Check sheet for the modelled part. Datum: model origin and axes. Units: mm. A direction names the side the tool comes from. Give positions to 0.01 mm unless a question says otherwise; leave off trailing zeros. Write each loop counter-clockwise with the first axis right and the second up, starting at its lowest first coordinate (ties: lowest second). Pieces come first, ordered by that corner, then holes. Notation, with made-up numbers: (30.5, 12) -> (41.5, 12) arc R24 ccw to (41.5, 22) -> close; hole circle Ø4 at (-13.75, 41.5). An arc over 180 degrees is marked (long way). Use a Markdown table: item, result. Add a question column.
1. Set-up check for faces 1 (the flat face through (5, 23, -37.008)), 2 (the flat face through (-1, -32.004, -31)): record each of +Z, -Z, +X, -X, +Y, -Y from which the full face is reachable in a straight line by a thin tool's end or side.
2. Scan lines: probe 1 along Y at (x, z) = (0, -49); probe 2 along X at (y, z) = (-7, -49.5); probe 3 along X at (y, z) = (0, -50). Record each from-to range of solid material in increasing order. Write a range as [from, to].
3. Cross-section at D-D (x = 31). Enter the section's corners in (y, z), then the cut area to 3 significant figures.
4. Cross-section at A-A (z = -51). Enter the section's corners in (x, y), then the cut area to 3 significant figures.
5. Cross-section at B-B (x = 0). Enter the section's corners in (y, z), then the cut area to 3 significant figures.
6. Release check for a two-part mould opening along X. For faces 3 (the flat face through (-43.002, -8, -38)), 4 (the flat face through (-1, -29, 0)), 5 (the cylindrical face through (-3.03, 23.07, -49.27)), 6 (the cylindrical face through (-33.39, -0.95, -40.33)) record: released by +X, released by -X, zero draft, split by the parting line, or undercut.
7. Cross-section at C-C (y = 0). Enter the section's corners in (x, z).
8. Gauge pin test, flat ends, axial feed: P1, Ø12, axis at x = -21.5, z = -25.5, coming from the +Y side; P2, Ø6, axis at x = 10.5, z = -24.5, coming from the +Y side; P3, Ø11, axis at x = 32.49, z = -47.02, coming from the -Y side. Record the tip position at first contact, or that the pin passes through.
from build123d import *

# Parameters (mm, degrees)
SKETCH1_W          = 86.0044
SKETCH1_H          = 62.992
SKETCH1_R          = 23.2665
EXTRUDE1_DEPTH     = 62.992
CUT_EXTRUDE1_DEPTH = 87.0044
SKETCH3_R          = 25.4
CUT_EXTRUDE2_DEPTH = 37.0078
FILLET1_R          = 1.524
HOLE1_D            = 13.4874
HOLE1_DEPTH        = 62.992


with BuildPart() as part:
    # Sketch1 → Extrude1 (new body)
    with BuildSketch(Plane.XY):
        with Locations((0, -0.508)):
            Rectangle(SKETCH1_W, SKETCH1_H)
        Circle(SKETCH1_R, mode=Mode.SUBTRACT)
    extrude(amount=-EXTRUDE1_DEPTH)

    # Sketch2 → Cut-Extrude1 (cut, through all)
    with BuildSketch(Plane(origin=(43.0022, 0, 0), x_dir=(0, 0, -1), z_dir=(1, 0, 0))):
        Polygon((0, 30.988), (37.592, 30.988), (0, -25.5016), align=None)
    extrude(amount=-CUT_EXTRUDE1_DEPTH, mode=Mode.SUBTRACT)

    # Sketch3 → Cut-Extrude2 (cut)
    with BuildSketch(Plane(origin=(0, 0, 0), x_dir=(-1, 0, 0), z_dir=(0, 0, -1))):
        with Locations(Location((0, 0, 0), (0, 0, 180))):  # turned: the seam where the file's is
            Circle(SKETCH3_R)
    extrude(amount=CUT_EXTRUDE2_DEPTH, mode=Mode.SUBTRACT)

    # Fillet1
    fillet1_edges = [part.edges().sort_by_distance(p)[0] for p in [
        (-25.4, 0, -37.0078),
    ]]
    fillet(fillet1_edges, radius=FILLET1_R)

    # Hole1
    with Locations(Plane(origin=(0, 30.988, 0), x_dir=(-1, 0, 0), z_dir=(0, 1, 0))):
        with Locations((32.512, -47.0154), (-32.4866, -47.0154)):
            Hole(HOLE1_D / 2, depth=HOLE1_DEPTH)

    # Sketch6 → Cut-Revolve1 (revolve, cut)
    with BuildSketch(Plane(origin=(0, 0, 0), x_dir=(-1, 0, 0), z_dir=(0, 1, 0)), mode=Mode.PRIVATE) as cut_revolve1_sk:
        Polygon((25.4, -34.671), (25.4, -35.433), (25.781, -35.052), align=None)
        Polygon((23.2665, -61.8745), (23.2665, -62.992), (24.384, -62.992), align=None)
    revolve(cut_revolve1_sk.sketch.rotate(Axis((0, 0, 17.508123997), (0, 0, -1)), 180), axis=Axis((0, 0, 17.508123997), (0, 0, -1)), mode=Mode.SUBTRACT)  # turned: the seam where the file's is


solid = part.part
Worked answers:
| question | item | result |
|---|---|---|
| 1 | face 1 | +Z |
| 1 | face 2 | +Z, -Z, +X, -X, -Y |
| 2 | probe 1 | y = [-32, -23.27], [23.27, 30.99] |
| 2 | probe 2 | x = [-43, -38.78], [-26.24, -22.19], [22.19, 26.22], [38.76, 43] |
| 2 | probe 3 | x = [-43, -38.56], [-26.46, -23.27], [23.27, 26.44], [38.53, 43] |
| 3 | outline | (-32, -62.99) -> (30.99, -62.99) -> (30.99, -53.59) -> (-32, -53.59) -> close; (-32, -40.44) -> (30.99, -40.44) -> (30.99, -37.59) -> (-25.5, 0) -> (-32, 0) -> close |
| 3 | area | 2,080 mm² |
| 4 | outline | (-43, -32) -> (-37.95, -32) -> (-37.95, 30.99) -> (-43, 30.99) -> close; (-27.07, -32) -> (27.05, -32) -> (27.05, 30.99) -> (-27.07, 30.99) -> close; (37.93, -32) -> (43, -32) -> (43, 30.99) -> (37.93, 30.99) -> close; hole circle Ø46.53 at (0, 0) |
| 4 | area | 2,350 mm² |
| 5 | outline | (-32, -62.99) -> (-24.38, -62.99) -> (-23.27, -61.87) -> (-23.27, -37.01) -> (-23.88, -37.01) arc R1.52 cw to (-25.4, -35.48) -> (-25.4, -35.43) -> (-25.78, -35.05) -> (-25.4, -34.67) -> (-25.4, -0.07) -> (-25.5, 0) -> (-32, 0) -> close; (23.27, -61.87) -> (24.38, -62.99) -> (30.99, -62.99) -> (30.99, -37.59) -> (25.4, -33.87) -> (25.4, -34.67) -> (25.78, -35.05) -> (25.4, -35.43) -> (25.4, -35.48) arc R1.52 cw to (23.88, -37.01) -> (23.27, -37.01) -> close |
| 5 | area | 679 mm² |
| 6 | face 3 | released by -X |
| 6 | face 4 | zero draft |
| 6 | face 5 | undercut |
| 6 | face 6 | undercut |
| 7 | outline | (-43, -62.99) -> (-24.38, -62.99) -> (-23.27, -61.87) -> (-23.27, -37.01) -> (-23.88, -37.01) arc R1.52 cw to (-25.4, -35.48) -> (-25.4, -35.43) -> (-25.78, -35.05) -> (-25.4, -34.67) -> (-25.4, -16.97) -> (-43, -16.97) -> close; (23.27, -61.87) -> (24.38, -62.99) -> (43, -62.99) -> (43, -16.97) -> (25.4, -16.97) -> (25.4, -34.67) -> (25.78, -35.05) -> (25.4, -35.43) -> (25.4, -35.48) arc R1.52 cw to (23.88, -37.01) -> (23.27, -37.01) -> close; hole circle Ø13.49 at (-32.51, -47.02); hole circle Ø13.49 at (32.49, -47.02) |
| 8 | P1 | stops at y = 21.83 |
| 8 | P2 | stops at y = -21.52 |
| 8 | P3 | passes through |
